Can you work these out from the drawing? Everything is in mm from the part's minimum corner. A direction names the side the tool comes from. Round coordinates to 2 decimals unless told otherwise and drop trailing zeros. Order: outer loops, then holes, each group sorted by start corner. A loop starts at its lowest first (then second) coordinate and runs counter-clockwise, first axis right, second up. Notation, with made-up numbers: M 40.5,75.5 L 74.5,75.5 A15 cw 74.5,100.5 Z; hole C 78,77 d4. An arc over 180 degrees is marked long. Write each question's results on one line, items separated by ' | '. Start each with the question number.
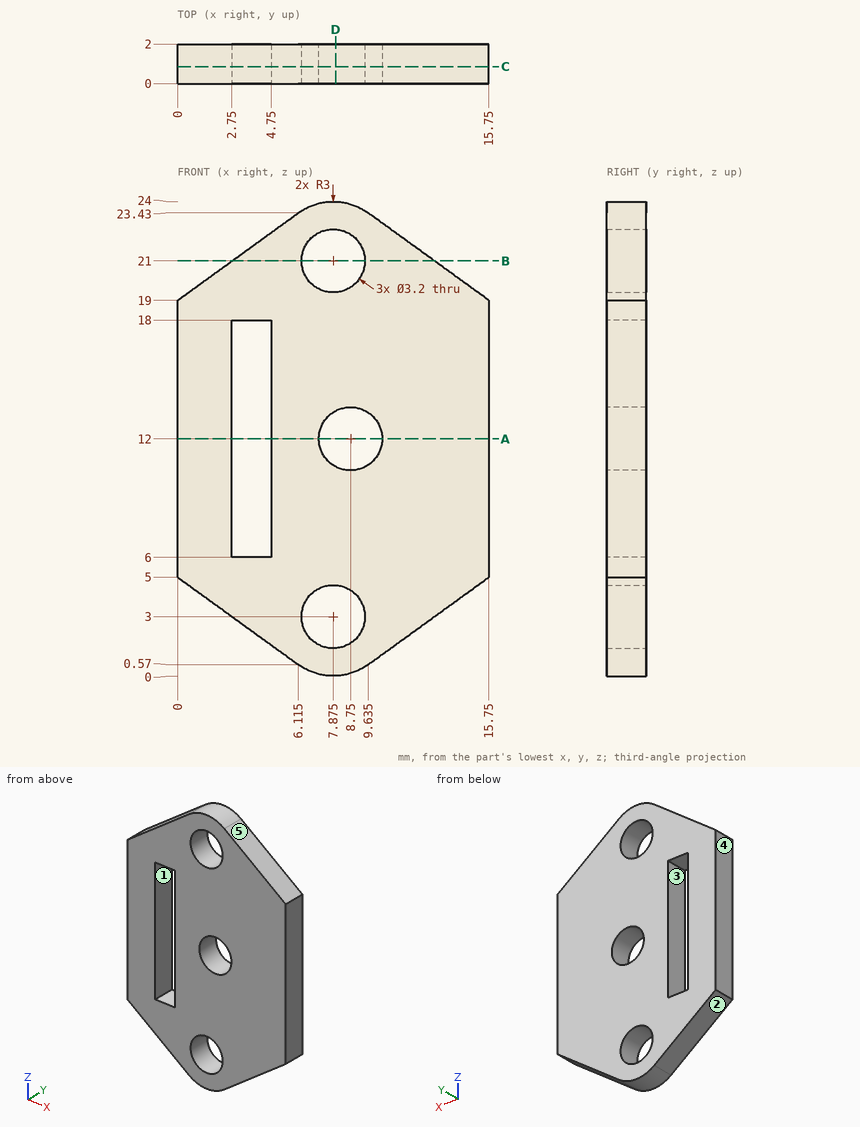
(1) I want a section at A-A on z = 12. Write out the boundary of the cut face in (x, y), and give its area (3 significant figures).
(2) I want a section at B-B on z = 21. Write out the boundary of the cut face in (x, y) (1 decimal).
(3) I want a section at D-D on x = 8. Write out the boundary of the cut face in (y, z) (1 decimal).
(4) On a 3-axis mill with a long thin cutter (end or side, diameter ignored), from which of +Z, -Z, +X, -X, +Y, -Y can I reach the whole of each face in a straight line? I mean the marked faces 1 and 2. Say none if no direction works.
(5) If we mould it in two halves opening along Z, with no side actions, what happens to the marked faces 3, 4 and 5? For each: pulls with the +Z half, pulls with the -Z half, needs draft (parallel to the pull), parting line crosses it, or undercut.
(6) I want a section at C-C on y = 0.85. Give the number of separate pieces and of enclosed holes in the cut face.
(7) Please list where these lines run through material, in increasing order: line 1 (Z direction, x = 8.5, y = 0.5) (1 decimal); line 2 (Z direction, x = 6.75, y = 0.95); line 3 (X direction, y = 1.45, z = 7.5).
(8) I'm going to push flat-ended pins straight in: pin 1 Ø4 at (x, z) = (7.875, 3) entering from +Y; pin 2 Ø1.9 at (x, z) = (7.875, 21) entering from -Y; pin 3 Ø0.6 at (x, y) = (3.5, 0.5) entering from -Z. Where does each tip first touch, or does it pass through?
Solutions:
1) outline: M 0,0 L 2.75,0 L 2.75,2 L 0,2 Z; M 4.75,0 L 7.15,0 L 7.15,2 L 4.75,2 Z; M 10.35,0 L 15.75,0 L 15.75,2 L 10.35,2 Z | area: 21.1 mm^2
2) outline: M 2.8,0 L 6.3,0 L 6.3,2 L 2.8,2 Z; M 9.5,0 L 13,0 L 13,2 L 9.5,2 Z
3) outline: M 0,0 L 2,0 L 2,1.4 L 0,1.4 Z; M 0,4.6 L 2,4.6 L 2,10.6 L 0,10.6 Z; M 0,13.4 L 2,13.4 L 2,19.4 L 0,19.4 Z; M 0,22.6 L 2,22.6 L 2,24 L 0,24 Z
4) face 1: +Y, -Y | face 2: -Z, -X, +Y, -Y
5) face 3: undercut | face 4: needs draft | face 5: pulls with the +Z half
6) separate pieces: 1 | enclosed holes: 4
7) line 1: 0.1 to 1.5, 4.5 to 10.4, 13.6 to 19.5, 22.5 to 23.9 | line 2: 0.22 to 1.86, 4.14 to 19.86, 22.14 to 23.78 | line 3: 0 to 2.75, 4.75 to 15.75
8) pin 1: y = 2 | pin 2: through | pin 3: z = 2.25
